Could you check a few things on this model? Use its own coordinates, in mm. A direction names the side the tool comes from. Round coordinates to 2 decimals unless told otherwise and drop trailing zeros. Order: outer loops, then holes, each group sorted by start corner. A loop starts at its lowest first (then second) coordinate and runs counter-clockwise, first axis right, second up. Notation, with made-up numbers: (11, 27) -> (46, 27) arc R16 ccw to (46, 50) -> close; hole circle Ø1 at (19.25, -32). An arc over 180 degrees is marked (long way). Put each result on its own line as item: value. Start each with the question number.
Autodesk Inventor part; units mm, degrees
ref_plane "YZ Plane" through (0, 0, 0) normal (1, 0, 0) x (0, 1, 0)
ref_plane "XZ Plane" through (0, 0, 0) normal (0, 1, 0) x (-1, 0, 0)
ref_plane "XY Plane" through (0, 0, 0) normal (0, 0, 1) x (1, 0, 0)
ref_plane "Arbeitsebene1" through (-19.3, 0, 0) normal (0, 0, 1) x (1, 0, 0)
sketch "Skizze1" plane through (-19.3, 0, 0) normal (0, 0, 1) x (1, 0, 0)
  line L0 (19.3, -32.4) -> (25.8, -32.4)
  line L1 (25.8, 0) -> (25.8, -32.4)
  line L2 (19.3, 0) -> (25.8, 0)
  line L3 (19.3, 0) -> (19.3, -32.4)
  circle A0 centre (22.9, -6.2) radius 1.75
  circle A1 centre (22.9, -26.2) radius 1.75
  line L4 (0, -32.4) -> (6.5, -32.4)
  line L5 (6.5, 0) -> (6.5, -32.4)
  line L6 (0, 0) -> (6.5, 0)
  line L7 (0, 0) -> (0, -32.4)
  circle A2 centre (2.9, -6.2) radius 1.75
  circle A3 centre (2.9, -26.2) radius 1.75
  line L8 (25.8, 0) -> (-19.2, 0)
  line L9 (-19.2, 0) -> (-19.2, -32.4)
  line L10 (-19.2, -32.4) -> (25.8, -32.4)
  line L11 (25.8, -32.4) -> (25.8, 0)
  dimension "d0" = 45
extrude "Extrusion1" add sketch "Skizze1" along normal blind 6
sketch "Skizze2" plane through (-38.5, -32.4, 0) normal (0, -1, 0) x (1, 0, 0)
  circle A0 centre (5.95, -6) radius 1.75
  line L0 (0, 0) -> (45, 0)
  line L1 (45, 0) -> (45, 6)
  line L2 (0, 6) -> (45, 6)
  line L3 (0, 0) -> (0, 6)
  line L4 (45, 0) -> (0, 0)
  line L5 (0, 0) -> (12, 0)
  line L6 (12, 0) -> (12, -12)
  line L7 (12, -12) -> (0, -12)
  line L8 (0, -12) -> (0, 0)
  circle A1 centre (5.95, -6) radius 1.6
  point P0 (38.5, 0)
  dimension "d3" = 12
  dimension "d4" = 12
  dimension "d5" = 3.2
extrude "Extrusion2" add sketch "Skizze2" against normal blind 6 contours L0 L6 L7 L8
sketch "Skizze3" plane through (-19.3, 0, 6) normal (0, 0, 1) x (1, 0, 0)
  circle A0 centre (22.9, -6.2) radius 1.75
  circle A1 centre (22.9, -26.2) radius 1.75
  circle A2 centre (2.9, -26.2) radius 1.75
  circle A3 centre (2.9, -6.2) radius 1.75
  point P0 (19.3, 0)
hole "Bohrung1" at (3.6, -26.2, 6) at (3.6, -6.2, 6) at (-16.4, -6.2, 6) at (-16.4, -26.2, 6) direction (0, 0, -1) diameter 3 end through all counterbore diameter 6.5 counterbore depth 3
sketch "Skizze4" plane through (-19.3, 0, 0) normal (0, 0, 1) x (1, 0, 0)
  arc A0 (25.8, -24.7328) -> (25.8, -27.6672) centre (22.9, -26.2) ccw
  line L0 (25.8, -24.7328) -> (25.8, -7.6672)
  arc A1 (25.8, -4.7328) -> (25.8, -7.6672) centre (22.9, -6.2) ccw
  line L1 (25.8, -4.7328) -> (25.8, 0)
  line L2 (25.8, 0) -> (-19.2, 0)
  line L3 (-19.2, 0) -> (-19.2, -32.4)
  line L4 (-19.2, -32.4) -> (25.8, -32.4)
  line L5 (25.8, -32.4) -> (25.8, -27.6672)
  circle A2 centre (2.9, -26.2) radius 3.25
  circle A3 centre (2.9, -6.2) radius 3.25
  circle A4 centre (22.9, -16.2) radius 1.4
  circle A5 centre (2.9, -16.2) radius 1.4
  circle A6 centre (12.9, -16.2) radius 1.4
  circle A7 centre (12.9, -6.2) radius 1.4
  circle A8 centre (12.9, -26.2) radius 1.4
  point P0 (19.3, 0)
  dimension "d15" = 2.8
  dimension "d16" = 2.8
  dimension "d17" = 20
  dimension "d18" = 0
  dimension "d19" = 2.8
  dimension "d20" = 10
  dimension "d21" = 2.8
  dimension "d22" = 2.8
hole "Bohrung2" at (-16.4, -16.2, 0) at (-6.4, -16.2, 0) at (-6.4, -26.2, 0) at (3.6, -16.2, 0) at (-6.4, -6.2, 0) direction (0, 0, 1) diameter 3 end through all counterbore diameter 6.5 counterbore depth 3
sketch "Skizze5" plane through (-38.5, -26.4, 0) normal (0, 1, 0) x (1, 0, 0)
  point P0 (38.5, 0)
sketch "Skizze6" plane through (-38.5, -32.4, 6) normal (0, -1, 0) x (1, 0, 0)
  circle A0 centre (5.95, -12) radius 1.75
  circle A1 centre (5.95, -12) radius 3.5
  point P0 (38.5, -6)
  dimension "d30" = 7
extrude "Extrusion3" cut sketch "Skizze6" against normal blind 4 contours A0 | A1
sketch "Skizze7" plane through (-19.3, 0, 6) normal (0, 0, 1) x (1, 0, 0)
  line L0 (25.8, -4.7328) -> (25.8, 0)
  circle A0 centre (22.9, -16.2) radius 1.5
  circle A1 centre (12.9, -16.2) radius 1.5
  circle A2 centre (2.9, -16.2) radius 1.5
  circle A3 centre (12.9, -26.2) radius 1.5
  circle A4 centre (12.9, -6.2) radius 1.5
  arc A5 (25.8, -24.7328) -> (25.8, -27.6672) centre (22.9, -26.2) ccw
  line L1 (25.8, -24.7328) -> (25.8, -7.6672)
  arc A6 (25.8, -4.7328) -> (25.8, -7.6672) centre (22.9, -6.2) ccw
  line L2 (25.8, -4.7328) -> (25.8, 0)
  line L3 (25.8, 0) -> (-19.2, 0)
  line L4 (-19.2, 0) -> (-19.2, -32.4)
  line L5 (-19.2, -32.4) -> (25.8, -32.4)
  line L6 (25.8, -32.4) -> (25.8, -27.6672)
  circle A7 centre (2.9, -26.2) radius 3.25
  circle A8 centre (2.9, -6.2) radius 3.25
  line L7 (0, 0) -> (0, -32.4)
  line L8 (25.8, 0) -> (0, 0)
  line L9 (0, 0) -> (0, 12)
  line L10 (0, 12) -> (25.8, 12)
  line L11 (25.8, 12) -> (25.8, 0)
  point P0 (19.3, 0)
  dimension "d34" = 12
extrude "Extrusion4" add sketch "Skizze7" against normal blind 6 contours L3 L9 L10 L11
sketch "Skizze8" plane through (-19.3, 0, 6) normal (0, 0, 1) x (1, 0, 0)
  circle A0 centre (22.9, 8.6709) radius 1.75
  circle A1 centre (2.9, 8.6709) radius 1.75
  circle A2 centre (22.9, -11.3291) radius 1.75
  circle A3 centre (2.9, -11.3291) radius 1.5
  line L0 (-3.15, 35.6) -> (-3.15, -57.8)
  point P0 (19.3, 14.8709)
hole "Bohrung3" at (3.6, 8.6709, 6) at (3.6, -11.3291, 6) at (-16.4, 8.6709, 6) at (-16.4, -11.3291, 6) direction (0, 0, -1) diameter 3 end through all counterbore diameter 6.5 counterbore depth 3
properties part number "Gripper_linear_arm_1"
1. If we section it at D-D, the plane z = 4: Count the separate pieces of the cut face and the enclosed holes in it, then the cut area to 3 significant figures.
2. I need wall thicknesses on L1, parallel to X at y = -16.2, z = 1.75; L2, parallel to Y at x = -6.4, z = 1.5; L3, parallel to X at y = -6.2, z = 4.4. Which ranges of each line are inside material? Lowest first, please.
3. Which directions (+Z, -Z, +X, -X, +Y, -Y) give clear straight access to the entire face, cutting with the end or side of a thin tool? Please do faces 5 (the face through (-13.152, 8.793, 4.479)), 6 (the face through (-33.9, -26.4, -4.6)), 7 (the face through (3, -18, 3)), 8 (the face through (-14.783, -5.53, 1.479)).
4. If we section it at B-B, the plane z = -6: Please give me the cut outline in (x, y).
5. Thinking about a two-plate mould opening in Y: for faces 1 (the face through (-38.5, -20, 1)), 2 (the face through (-32, -28.4, -4)), 3 (the face through (-4.422, -28.779, 1.521)), 4 (the face through (-29, 0, 3)), which applies, +Y half, -Y half, draft (parallel to the pull), parting line (faces both ways), or undercut?
6. If we section it at C-C, the plane x = -32.55: Please give me the cut outline in (y, z), then the cut area to 3 significant figures.
7. If we section it at A-A, the plane x = -6.4: Please give me the cut outline in (y, z), then the cut area to 3 significant figures.
8. For pin 1 Ø4 at (x, y) = (-16.4, 8.67) entering from +Z; pin 2 Ø6 at (x, y) = (3.6, -6.2) entering from -Z; pin 3 Ø2.5 at (x, y) = (3.6, 8.67) entering from -Z; pin 4 Ø5 at (y, z) = (9, 2.5) entering from -X, each with a flat end and sliding along its axis, tell me the tip position at first contact or that it passes through.
Results below:
1. separate pieces: 2
1. enclosed holes: 7
1. area: 1,480 mm2
2. L1: -38.5 to -19.65, -13.15 to -9.65, -3.15 to 0.35
2. L2: -32.4 to -29.45, -22.95 to -19.45, -12.95 to -9.45, -2.95 to 12
2. L3: -38.5 to -19.65, -13.15 to -7.9, -4.9 to 0.35
3. face 5: +Z
3. face 6: -Z, +X, -X, +Y
3. face 7: -Z
3. face 8: +Z, -Z
4. outline: (-38.5, -32.4) -> (-36.05, -32.4) -> (-36.05, -28.4) -> (-34.3, -28.4) -> (-34.3, -26.4) -> (-38.5, -26.4) -> close; (-30.8, -28.4) -> (-29.05, -28.4) -> (-29.05, -32.4) -> (-26.5, -32.4) -> (-26.5, -26.4) -> (-30.8, -26.4) -> close
5. face 1: draft
5. face 2: -Y half
5. face 3: undercut
5. face 4: +Y half
6. outline: (-32.4, -12) -> (-26.4, -12) -> (-26.4, -7.75) -> (-28.4, -7.75) -> (-28.4, -9.5) -> (-32.4, -9.5) -> close; (-32.4, -2.5) -> (-28.4, -2.5) -> (-28.4, -4.25) -> (-26.4, -4.25) -> (-26.4, 0) -> (0, 0) -> (0, 6) -> (-32.4, 6) -> close
6. area: 231 mm2
7. outline: (-32.4, 0) -> (-29.45, 0) -> (-29.45, 3) -> (-27.7, 3) -> (-27.7, 6) -> (-32.4, 6) -> close; (-24.7, 3) -> (-22.95, 3) -> (-22.95, 0) -> (-19.45, 0) -> (-19.45, 3) -> (-17.7, 3) -> (-17.7, 6) -> (-24.7, 6) -> close; (-14.7, 3) -> (-12.95, 3) -> (-12.95, 0) -> (-9.45, 0) -> (-9.45, 3) -> (-7.7, 3) -> (-7.7, 6) -> (-14.7, 6) -> close; (-4.7, 3) -> (-2.95, 3) -> (-2.95, 0) -> (12, 0) -> (12, 6) -> (-4.7, 6) -> close
7. area: 181 mm2
8. pin 1: z = 3
8. pin 2: z = 0
8. pin 3: through
8. pin 4: x = -19.3
